Design review of the part built by this model. Coordinates are the model's own, in mm. A direction names the side the tool comes from. Give positions to 0.01 mm unless a question says otherwise; leave off trailing zeros. Write each loop counter-clockwise with the first axis right and the second up, starting at its lowest first coordinate (ties: lowest second). Pieces come first, ordered by that corner, then holes.
Autodesk Inventor part; units mm, degrees
ref_plane "YZ Plane" through (0, 0, 0) normal (1, 0, 0) x (0, 1, 0)
ref_plane "XZ Plane" through (0, 0, 0) normal (0, 1, 0) x (-1, 0, 0)
ref_plane "XY Plane" through (0, 0, 0) normal (0, 0, 1) x (1, 0, 0)
sketch "草图1" plane through (0, 0, 0) normal (0, 0, 1) x (1, 0, 0)
  circle A0 centre (0, 41) radius 4.25
  circle A1 centre (0, 41) radius 4.25
  line L0 (0, 41) -> (-2.75, 36.2369)
  line L1 (0, 41) -> (5.5, 41) construction
  line L2 (0, 41) -> (-5.5, 41)
  line L3 (0.7501, 46.4486) -> (42.3728, 40.7189)
  line L4 (-15, 3) -> (-15, 6)
  line L5 (-15, 6) -> (-18, 6)
  line L6 (-18, 6) -> (-18, -8)
  line L7 (-4, -8) -> (-18, -8)
  line L8 (-4, -6) -> (-4, -8)
  line L9 (-4, -6) -> (4, -6)
  line L10 (4, -6) -> (4, -8)
  line L11 (18, -8) -> (4, -8)
  line L12 (18, 6) -> (18, -8)
  line L13 (18, 6) -> (15, 6)
  line L14 (15, 6) -> (15, 3)
  line L15 (15, 3) -> (13.5, 3)
  line L16 (13.5, 3) -> (13.5, 2)
  line L17 (13.5, 2) -> (15, 2)
  line L18 (15, 2) -> (15, -2)
  line L19 (15, -2) -> (-15, -2)
  line L20 (-15, -2) -> (-15, 2)
  line L21 (-15, 2) -> (-13.5, 2)
  line L22 (-13.5, 2) -> (-13.5, 3)
  line L23 (-13.5, 3) -> (-15, 3)
  line L24 (-18, -8) -> (18, -8)
  line L25 (18, -8) -> (18, -12)
  line L26 (18, -12) -> (-18, -12)
  line L27 (-18, -12) -> (-18, -8)
  line L28 (18, -12) -> (42.3728, -12)
  line L29 (42.3728, -12) -> (42.3728, 40.7189)
  line L30 (18, -8) -> (38, -8)
  line L31 (38, -8) -> (38, 37.0777)
  line L32 (0.2288, 35.5048) -> (38, 37.0777)
  arc A2 (-2.75, 36.2369) -> (0.2288, 35.5048) centre (0, 41) ccw
  arc A3 (0.7501, 46.4486) -> (-5.5, 41) centre (0, 41) ccw
  point P0 (0, 0)
  point P1 (-4.25, 41)
  point P2 (-2.125, 37.3194)
  dimension "d1" = 120
  dimension "d2" = 4
  dimension "d3" = 20
extrude "拉伸1" add sketch "草图1" against normal blind 50 contours A0 L2 A3 L3 L29 L28 L25 L30 L31 L32 A2 L0 | L26 L27 L7 L24 L11 L25
fillet "圆角1" radius 5 2 edges at (38, 37.0777, -25) (42.3728, 40.7189, -25)
fillet "圆角2" radius 5 2 edges at (38, -8, -25) (42.3728, -12, -25)
sketch "草图2" plane through (-18, -12, -50) normal (0, -1, 0) x (1, 0, 0)
  line L0 (0, 50) -> (55.3728, 50)
  line L1 (0, 50) -> (0, 0)
  line L2 (55.3728, 0) -> (0, 0)
  point P0 (18, 50)
  point P1 (7, 42)
  point P2 (7, 8)
  point P3 (29, 42)
  point P4 (29, 8)
  dimension "d8" = 8
  dimension "d9" = 7
  dimension "d10" = 8
  dimension "d11" = 22
hole "孔1" at (-11, -12, -8) at (-11, -12, -42) at (11, -12, -8) at (11, -12, -42) direction (0, 1, 0) diameter 3.242 depth 4 countersink diameter 4 countersink angle 90
sketch "草图3" plane through (-18, -12, -50) normal (0, -1, 0) x (1, 0, 0)
  line L0 (0, 50) -> (0, 0)
  line L1 (0, 35) -> (55, 35)
  line L2 (55, 35) -> (55, 15)
  line L3 (55, 15) -> (0, 15)
  line L4 (0, 15) -> (0, 35)
  line L5 (0, 50) -> (55.3728, 50)
  point P0 (18, 50)
  point P1 (0, 15)
  dimension "d19" = 55
  dimension "d20" = 20
  dimension "d21" = 15
extrude "拉伸2" add sketch "草图3" along normal blind 20
properties part number "链接板2"
(1) Consider section C-C, the plane z = -37.5. Give the boundary of the cut face in (x, y), then the cut area to 3 significant figures.
Resolved:
outline: (-18, -12) - (37.37, -12) arc R5 ccw to (42.37, -7) - (42.37, 36.36) arc R5 ccw to (38.05, 41.31) - (0.75, 46.45) arc R5.5 ccw to (-5.5, 41) - (-4.25, 41) arc R4.25 cw (long way) to (-2.13, 37.32) - (-2.75, 36.24) arc R5.5 ccw to (0.23, 35.5) - (32.79, 36.86) arc R5 cw to (38, 31.87) - (38, -3) arc R5 cw to (33, -8) - (-18, -8) - close
area: 733 mm2
(2) Consider section A-A, the plane z = -8. Give the boundary of the cut face in (x, y), then the cut area to 3 significant figures.
Resolved:
outline: (-18, -12) - (-13, -12) - (-12.62, -11.62) - (-12.62, -8) - (-18, -8) - close; (-9.38, -11.62) - (-9, -12) - (9, -12) - (9.38, -11.62) - (9.38, -8) - (-9.38, -8) - close; (-5.5, 41) - (-4.25, 41) arc R4.25 cw (long way) to (-2.13, 37.32) - (-2.75, 36.24) arc R5.5 ccw to (0.23, 35.5) - (32.79, 36.86) arc R5 cw to (38, 31.87) - (38, -3) arc R5 cw to (33, -8) - (12.62, -8) - (12.62, -11.62) - (13, -12) - (37.37, -12) arc R5 ccw to (42.37, -7) - (42.37, 36.36) arc R5 ccw to (38.05, 41.31) - (0.75, 46.45) arc R5.5 ccw to start
area: 707 mm2
(3) To check wall thickness, follow L1, parallel to Y at x = 0, z = -26.5; L2, parallel to Z at x = 11, y = -9; L3, parallel to Y at x = 0, z = -12.5. State the ranges of each line that lie inside material, in increasing order.
Resolved:
L1: y = -32 to -8, 35.5 to 36.75, 45.25 to 46.5
L2: z = -50 to -43.62, -40.38 to -9.62, -6.38 to 0
L3: y = -12 to -8, 35.5 to 36.75, 45.25 to 46.5
(4) Consider section D-D, the plane x = 11. Give the boundary of the cut face in (y, z), then the cut area to 3 significant figures.
Resolved:
outline: (-32, -35) - (-12, -35) - (-12, -40) - (-11.62, -40.38) - (-8, -40.38) - (-8, -9.62) - (-11.62, -9.62) - (-12, -10) - (-12, -15) - (-32, -15) - close; (-12, -50) - (-8, -50) - (-8, -43.62) - (-11.62, -43.62) - (-12, -44) - close; (-12, -6) - (-11.62, -6.38) - (-8, -6.38) - (-8, 0) - (-12, 0) - close; (35.95, -50) - (45.04, -50) - (45.04, 0) - (35.95, 0) - close
area: 1,030 mm2
(5) Clearance check with flat-ended pins moving along their axes: P1, Ø4, axis at x = -6.5, z = -23.5, coming from the +Y side; P2, Ø12, axis at x = 28, y = 36, coming from the -Z side; P3, Ø5, axis at x = 19, z = -22, coming from the +Y side; P4, Ø3, axis at x = 11, z = -42, coming from the -Y side. State where each tip first meets the part, or that it passes through.
Resolved:
P1: stops at y = 44.16
P2: stops at z = -50
P3: stops at y = 44.28
P4: stops at y = 35.89
(6) Consider section B-B, the plane x = 30.5. Give the boundary of the cut face in (y, z), then the cut area to 3 significant figures.
Resolved:
outline: (-32, -35) - (-12, -35) - (-12, -50) - (-8, -50) - (-8, 0) - (-12, 0) - (-12, -15) - (-32, -15) - close; (36.77, -50) - (42.35, -50) - (42.35, 0) - (36.77, 0) - close
area: 879 mm2
(7) Tool access review of faces 5 (the face through (9.9, -9.79, -40.81)), 6 (the face through (10, -22, -35)), 7 (the face through (16.282, 36.173, -24.65)): name each direction out of +Z, -Z, +X, -X, +Y, -Y from which nothing blocks a thin tool from reaching the whole face with its end or side.
Resolved:
face 5: -Y
face 6: -Z, +X, -X, -Y
face 7: +Z, -Z
(8) Mouldability with a two-part tool opening along Y and no side actions: class faces 1 (the face through (9, -32, -25)), 2 (the face through (9.9, -9.79, -6.81)), 3 (the face through (41.11, 39.68, -25.35)), 4 (the face through (7, -8, -25)) as pulls with the +Y half, pulls with the -Y half, needs draft (parallel to the pull), parting line crosses it, or undercut.
Resolved:
face 1: pulls with the -Y half
face 2: needs draft
face 3: pulls with the +Y half
face 4: undercut
